```python
from build123d import *

# Parameters (mm, degrees)
F3_W      = 38.1
F3_H      = 38.1
F4_DEPTH  = 38.1
F6_DEPTH  = 38.1
F8_DEPTH  = 38.1
F10_DEPTH = 38.1


with BuildPart() as f4:
    # F3 (on Front) → F4 (new body)
    with BuildSketch(Plane.XZ):
        with Locations((19.05, 19.05)):
            Rectangle(F3_W, F3_H)
    extrude(amount=F4_DEPTH)

    # F5 (on offset) → F6 (cut)
    with BuildSketch(Plane.XZ.offset(38.1)):
        Polygon((0, 26.67), (0, 7.174831), (5.08, 7.174831), (12.7, 10.795), (12.7, 26.67), align=None)
        Polygon((26.67, 8.89), (19.05, 0), (38.1, 0), (38.1, 26.67), (26.67, 26.67), align=None)
    extrude(amount=-F6_DEPTH, mode=Mode.SUBTRACT)

    # F7 (on offset) → F8 (cut)
    with BuildSketch(Plane.YZ.offset(38.1)):
        Polygon((-38.1, 26.67), (-38.1, 6.268343), (-33.02, 6.268343), (-25.4, 10.795), (-25.4, 26.67), align=None)
        Polygon((-19.05, 0), (0, 0), (0, 26.67), (-11.43, 26.67), (-11.43, 8.89), align=None)
    extrude(amount=-F8_DEPTH, mode=Mode.SUBTRACT)

    # F9 (on offset) → F10 (cut)
    with BuildSketch(Plane.XY.offset(38.1)):
        Polygon((7.62, -29.21), (7.62, -38.1), (22.86, -38.1), (16.51, -29.21), align=None)
        Polygon((19.05, -7.62), (7.62, -7.62), (7.62, -20.32), (17.297857, -20.32), (22.396552, -17.78), (24.747821, -15.24), (24.407931, -10.16), align=None)
        Polygon((38.1, -38.1), (38.1, -16.605278), (30.532379, -21.050278), (27.94, -24.860278), align=None)
        Polygon((38.1, 0), (28.555734, 0), (34.945868, -3.50978), (38.1, -7.62), align=None)
    extrude(amount=-F10_DEPTH, mode=Mode.SUBTRACT)


solid = f4.part
```
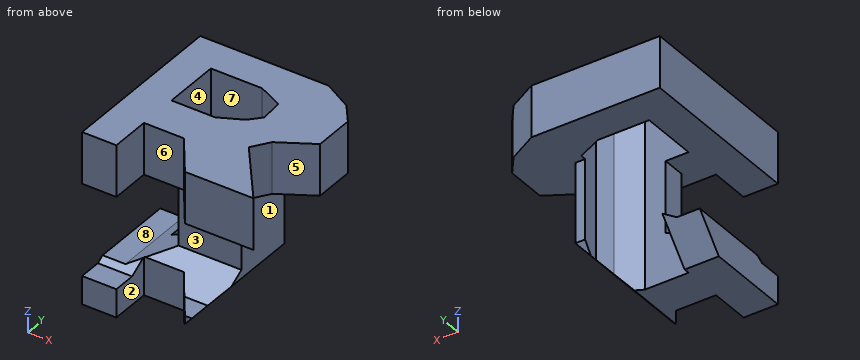
Here's how the part is built. I have some questions about the finished solid (model axes, mm). Face numbers are marked on the shaded views. A direction names the side the tool comes from. Give positions to 0.01 mm unless a question says otherwise; leave off trailing zeros. Order: outer loops, then holes, each group sorted by start corner. A loop starts at its lowest first (then second) coordinate and runs counter-clockwise, first axis right, second up. Notation, with made-up numbers: M 70.25,30 L 78.25,30 A29 ccw 78.25,59 Z; hole C 16,84.5 d2. An arc over 180 degrees is marked long. Use a Markdown table: item, result. Add a question column.
1. Suppose I cut it at A-A (x = 3.5). List the corners of the cut face in (y, z) for me, and give its area (3 significant figures).
2. Suppose I cut it at D-D (y = -27). List the corners of the cut face in (x, z) for me.
3. Suppose I cut it at C-C (y = -34). List the corners of the cut face in (x, z) for me, and give its area (3 significant figures).
4. If we mould it in two halves opening along Y, with no side actions, what happens to the marked faces 6, 7 and 8? For each: +Y half, -Y half, draft (parallel to the pull), parting line (faces both ways), or undercut.
5. For pin 1 Ø1.7 at (x, z) = (25.5, 20.5) entering from +Y; pin 2 Ø9 at (x, z) = (13, 32) entering from -Y; pin 3 Ø6 at (x, y) = (9, -22) entering from -Z; pin 4 Ø12 at (x, z) = (14, 7.5) entering from +Y, each with a flat end and sliding along its axis, tell me the tip position at first contact or that it passes through.
6. On a 3-axis mill with a long thin cutter (end or side, diameter ignored), from which of +Z, -Z, +X, -X, +Y, -Y can I reach the whole of each face in a straight line? I mean the marked faces 1, 2, 3, 4 and 5. Say none if no direction works.
7. I need wall thicknesses on probe 1 along Y at (x, z) = (8, 31); probe 2 along Z at (x, y) = (6, -26); probe 3 along Z at (x, y) = (27, -26.5). Which ranges of each line are inside material? Lowest first, please. Write a range as from..to.
8. Suppose I cut it at B-B (z = 33). List the corners of the cut face in (x, y) for me, and give its area (3 significant figures).
Results list:
| question | item | result |
|---|---|---|
| 1 | outline | M -38.1,0 L -19.05,0 L -12.9,7.17 L -31.49,7.17 L -33.02,6.27 L -38.1,6.27 Z; M -38.1,26.67 L 0,26.67 L 0,38.1 L -38.1,38.1 Z |
| 1 | area | 589 mm² |
| 2 | outline | M 0,0 L 19.05,0 L 26.67,8.89 L 26.67,9.84 L 10.7,9.84 L 5.08,7.17 L 0,7.17 Z; M 0,26.67 L 29.58,26.67 L 29.58,38.1 L 0,38.1 Z |
| 3 | outline | M 0,0 L 7.62,0 L 7.62,6.27 L 0,6.27 Z; M 0,26.67 L 7.62,26.67 L 7.62,38.1 L 0,38.1 Z; M 19.93,1.03 L 24.42,6.27 L 19.93,6.27 Z; M 19.93,26.67 L 34.95,26.67 L 34.95,38.1 L 19.93,38.1 Z |
| 3 | area | 318 mm² |
| 4 | face 6 | -Y half |
| 4 | face 7 | undercut |
| 4 | face 8 | draft |
| 5 | pin 1 | stops at y = -11.43 |
| 5 | pin 2 | stops at y = -30.6 |
| 5 | pin 3 | stops at z = 0 |
| 5 | pin 4 | stops at y = -18.97 |
| 6 | face 1 | -Z, +X, +Y, -Y |
| 6 | face 2 | +Z, -Z, -Y |
| 6 | face 3 | +X, -X, -Y |
| 6 | face 4 | +Z, -Z |
| 6 | face 5 | +Z, -Z, +X |
| 7 | probe 1 | y = -29.21..-20.32, -7.62..0 |
| 7 | probe 2 | z = 0..7.61, 26.67..38.1 |
| 7 | probe 3 | z = 26.67..38.1 |
| 8 | outline | M 0,-38.1 L 7.62,-38.1 L 7.62,-29.21 L 16.51,-29.21 L 22.86,-38.1 L 38.1,-38.1 L 27.94,-24.86 L 30.53,-21.05 L 38.1,-16.61 L 38.1,-7.62 L 34.95,-3.51 L 28.56,0 L 0,0 Z; hole M 7.62,-20.32 L 17.3,-20.32 L 22.4,-17.78 L 24.75,-15.24 L 24.41,-10.16 L 19.05,-7.62 L 7.62,-7.62 Z |
| 8 | area | 1,000 mm² |
